The drawing under review shows one solid part. Ordinate dimensions are in mm from its lowest x, y, z. A direction names the side the tool comes from. Give positions to 0.01 mm unless a question says otherwise; leave off trailing zeros. Write each loop counter-clockwise with the first axis right and the second up, starting at its lowest first coordinate (ties: lowest second). Pieces come first, ordered by that corner, then holes. Notation, with made-up numbers: (-34.75, 66.5) -> (-17.75, 66.5) arc R28 ccw to (-17.75, 104.5) -> close; hole circle Ø9 at (-24.75, 30.5). An arc over 180 degrees is marked (long way). Answer as a JSON object with one key per item and string values.
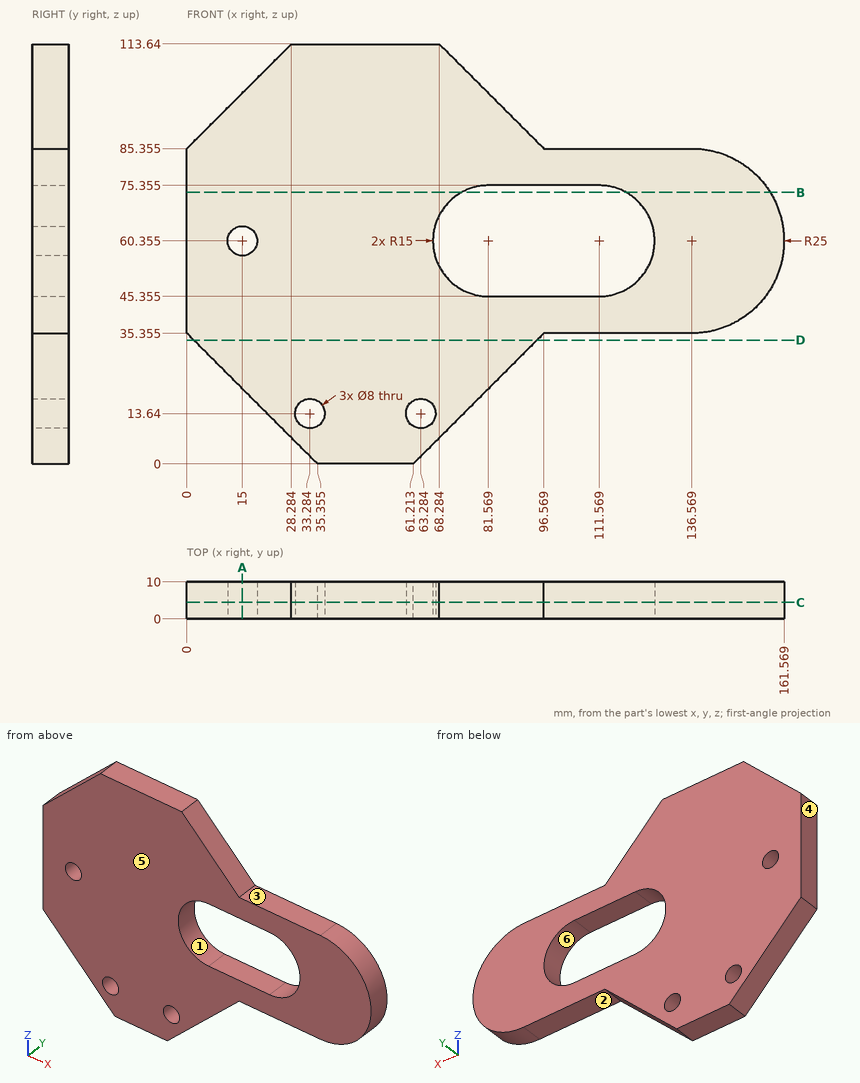
(1) The part is to be moulded in two halves that separate along X. For the marked faces 4, 5 and 6, say which applies: +X half, -X half, draft (parallel to the pull), parting line (faces both ways), or undercut.
Here are the results:
{"face 4": "-X half", "face 5": "draft", "face 6": "undercut"}
(2) For the marked faces 1, 2 and 3, list the 3-axis set-ups (+Z, -Z, +X, -X, +Y, -Y) from which the entire face can be reached by the end or side of a thin tool; tool diameter is ignored.
Here are the results:
{"face 1": "+Y, -Y", "face 2": "-Z, +X, +Y, -Y", "face 3": "+Z, +X, +Y, -Y"}
(3) We need section C-C, the plane y = 4.5. State the section outline as (x, z) points (1 decimal), then the cut area to 3 significant figures.
Here are the results:
{"outline": "(0, 35.4) -> (35.4, 0) -> (61.2, 0) -> (96.6, 35.4) -> (136.6, 35.4) arc R25 ccw to (136.6, 85.4) -> (96.6, 85.4) -> (68.3, 113.6) -> (28.3, 113.6) -> (0, 85.4) -> close; hole circle Ø8 at (15, 60.4); hole circle Ø8 at (33.3, 13.6); hole circle Ø8 at (63.3, 13.6); hole (81.6, 45.4) -> (111.6, 45.4) arc R15 ccw to (111.6, 75.4) -> (81.6, 75.4) arc R15 ccw to start", "area": "10,100 mm²"}
(4) Clearance check with flat-ended pins moving along their axes: pin 1 (3 mm diameter, centred on y = 3.5, z = 78.5, fed in from +X); pin 2 (1.5 mm diameter, centred on y = 6, z = 44, fed in from +X); pin 3 (5 mm diameter, centred on x = 55, y = 2.5, fed in from -Z); pin 4 (2 mm diameter, centred on y = 2.5, z = 33.5, fed in from +X) (1 decimal). State where each tip first meets the part, or that it passes through.
Here are the results:
{"pin 1": "stops at x = 155.22", "pin 2": "stops at x = 156.1", "pin 3": "stops at z = 0", "pin 4": "stops at x = 95.7"}
(5) We need section D-D, the plane z = 33.5. State the section outline as (x, y) points (1 decimal).
Here are the results:
{"outline": "(1.9, 0) -> (94.7, 0) -> (94.7, 10) -> (1.9, 10) -> close"}
(6) For line 1 along X through (y, z) = (4.5, 15) (1 decimal); line 2 along X through (y, z) = (8.5, 13.5) (1 decimal); line 3 along Z through (x, y) = (92, 4.75) (1 decimal), list the stretches that pass through material, from the lowest coordinate up.
Here are the results:
{"line 1": "x = 20.4 to 29.5, 37 to 59.5, 67 to 76.2", "line 2": "x = 21.9 to 29.3, 37.3 to 59.3, 67.3 to 74.7", "line 3": "z = 30.8 to 45.4, 75.4 to 89.9"}
(7) We need section A-A, the plane x = 15. State the section outline as (y, z) points (1 decimal), then the cut area to 3 significant figures.
Here are the results:
{"outline": "(0, 20.4) -> (10, 20.4) -> (10, 56.4) -> (0, 56.4) -> close; (0, 64.4) -> (10, 64.4) -> (10, 100.4) -> (0, 100.4) -> close", "area": "720 mm²"}
(8) We need section B-B, the plane z = 73.5. State the section outline as (x, y) points (1 decimal), then the cut area to 3 significant figures.
Here are the results:
{"outline": "(0, 0) -> (74.3, 0) -> (74.3, 10) -> (0, 10) -> close; (118.8, 0) -> (157.8, 0) -> (157.8, 10) -> (118.8, 10) -> close", "area": "1,130 mm²"}
